Source: CAD feature listing. Evaluate the final solid. Frame: model axes, mm. A direction names the side the tool comes from. Give positions to 0.01 mm unless a question says otherwise; leave off trailing zeros. Order: outer loops, then holes, each group sorted by start corner. A loop starts at its lowest first (then second) coordinate and runs counter-clockwise, first axis right, second up.
1) First-contact query: P1, Ø0.6, axis at y = 5, z = 1.5, coming from the -X side; P2, Ø4, axis at x = 2, y = 9.5, coming from the +Z side; P3, Ø0.6, axis at x = 3.5, z = 1.5, coming from the -Y side; P4, Ø1, axis at y = -3.5, z = 1.5, coming from the +X side. Flat tips, straight axial feed; report the tip coordinate or a pass-through.
2) Section C-C, the plane x = 3.75. Return loops of the section in (y, z) (3 decimals).
3) Access query for faces 4 (the face through (-9.248, 14.287, 1.014)), 5 (the face through (2.5, -3, 1)), 6 (the face through (-4, 0, 1)). Directions: +Z, -Z, +X, -X, +Y, -Y. A direction counts if a zero-diameter tool reaches every point of the face in a straight line with its end or side. Return the directions, or none.
4) Section B-B, the plane y = 9. Return loops of the section in (x, z).
5) Material intervals for line 1 (Y direction, x = -7.5, z = 0.75); line 2 (Y direction, x = 0, z = 0.8); line 3 (X direction, y = -3.25, z = 1.9), sorted ascending.
6) Draft query along X for faces 1 (the face through (0.436, 6.846, 0.986)), 2 (the face through (-8.05, 13.01, 0.99)), 3 (the face through (0, -5, 1)). Return one class per face: released by +X, released by -X, zero draft, split by the parting line, or undercut.
```python
from build123d import *

# Parameters (mm, degrees)
F0_R     = 0.75
F0_W     = 5
F0_H     = 5
F1_DEPTH = 2
F2_R     = 2.49999


# Not quite as in the source:
# - a fillet or chamfer is up to 0.001 mm smaller than in the source, because OpenCascade refuses the exact size


with BuildPart() as f1:
    # F0 (on Top) → F1 (new body)
    with BuildSketch(Plane.XY):
        Polygon((-5, 0), (-2.5, 0), (2.5, 0), (5, 0), (-5, 15), (-10, 15), (-10, 10), (-5, 10), align=None)
        with Locations((-7.5, 12.5)):
            Circle(F0_R, mode=Mode.SUBTRACT)
        with Locations((0, -2.5)):
            Rectangle(F0_W, F0_H)
    extrude(amount=F1_DEPTH)

    # F2 (radius 2.5 in the source; OpenCascade refuses exactly that, so slightly less here)
    f2_edges = [f1.edges().sort_by_distance(p)[0] for p in [
        (-10, 15, 1),
        (-10, 10, 1),
        (-5, 15, 1),
        (-5, 10, 1),
    ]]
    fillet(f2_edges, radius=F2_R)


solid = f1.part
```
From the geometry:
1. P1: stops at x = -5
1. P2: passes through
1. P3: stops at y = 0
1. P4: stops at x = 2.5
2. outline: (0, 0) - (1.875, 0) - (1.875, 2) - (0, 2) - close
3. face 4: +Z, -Z, -X, +Y
3. face 5: +Z, -Z, +X, -Y
3. face 6: +Z, -Z, -X, -Y
4. outline: (-5.5, 0) - (-1, 0) - (-1, 2) - (-5.5, 2) - close
5. line 1: y = 10 to 11.75, 13.25 to 15
5. line 2: y = -5 to 7.5
5. line 3: x = -2.5 to 2.5
6. face 1: released by +X
6. face 2: undercut
6. face 3: zero draft
